The listing builds one solid part. Answer for the finished solid, in the listing's coordinates (mm). A direction names the side the tool comes from. Round coordinates to 2 decimals unless told otherwise and drop trailing zeros. Loops run counter-clockwise (first coordinate to the right, second up) from the corner with the lowest first, then second, coordinate; pieces in that order, holes last. Notation, with made-up numbers: (23.25, 47) -> (36.25, 47) arc R12 ccw to (36.25, 59) -> close; hole circle Ø8 at (51.5, 2). An arc over 180 degrees is marked (long way). Write each question's results on one line, items separated by ' | '. Start each with the question number.
from build123d import *

# Parameters (mm, degrees)
SKETCH1_W           = 44
SKETCH1_H           = 44
SKETCH1_R           = 2.25
SKETCH1_R_2         = 12
BOSS_EXTRUDE1_DEPTH = 5
SKETCH2_W           = 50
SKETCH2_H           = 44
SKETCH2_R           = 2.5
BOSS_EXTRUDE2_DEPTH = 5
BOSS_EXTRUDE3_DEPTH = 15
CHAMFER1_SIZE       = 7
CHAMFER2_SIZE       = 2
SKETCH4_W           = 50
SKETCH4_H           = 10.75
BOSS_EXTRUDE4_DEPTH = 10
CHAMFER3_SIZE       = 9
CHAMFER4_SIZE       = 2


with BuildPart() as part:
    # Sketch1 → Boss-Extrude1 (new body)
    with BuildSketch(Plane.XY):
        Rectangle(SKETCH1_W, SKETCH1_H)
        with Locations((15.5, 15.5)):
            Circle(SKETCH1_R, mode=Mode.SUBTRACT)
        with Locations((15.5, -15.5)):
            Circle(SKETCH1_R, mode=Mode.SUBTRACT)
        with Locations((-15.5, -15.5)):
            Circle(SKETCH1_R, mode=Mode.SUBTRACT)
        with Locations((-15.5, 15.5)):
            Circle(SKETCH1_R, mode=Mode.SUBTRACT)
        Circle(SKETCH1_R_2, mode=Mode.SUBTRACT)
    extrude(amount=BOSS_EXTRUDE1_DEPTH)

    # Sketch2 → Boss-Extrude2 (add)
    with BuildSketch(Plane.ZY.offset(22)):
        with Locations((25, 0)):
            Rectangle(SKETCH2_W, SKETCH2_H)
        with Locations(Location((44, 0, 0), (0, 0, 270))):
            Circle(SKETCH2_R, mode=Mode.SUBTRACT)
        with Locations(Location((24, 0, 0), (0, 0, 270))):
            Circle(SKETCH2_R, mode=Mode.SUBTRACT)
    extrude(amount=BOSS_EXTRUDE2_DEPTH)

    # Sketch3 → Boss-Extrude3 (add, symmetric)
    with BuildSketch(Plane(origin=(0, 0, 0), x_dir=(1, 0, 0), z_dir=(0, 1, 0))):
        Polygon((-14, -5), (-22, -13), (-22, -5), align=None)
    extrude(amount=BOSS_EXTRUDE3_DEPTH, both=True)

    # Chamfer1
    # the kernel refuses this chamfer: 7 mm, written as the material it takes off along each edge
    with BuildSketch(Plane(origin=(-1.270818641, -15, -7.729181359), x_dir=(-0.7068394360706735, -0.02749587661058637, -0.7068394360706736), z_dir=(-0.7071067811865477, 0, 0.7071067811865475))) as chamfer1_piece_1_section:
        Polygon((CHAMFER1_SIZE * 0.999621916911, -CHAMFER1_SIZE * 0.0274958766106), (-CHAMFER1_SIZE * 0.0274958766106, -CHAMFER1_SIZE * 0.999621916911), (0, 0), align=None)
    chamfer1_piece_1 = extrude(amount=47.317270331, mode=Mode.PRIVATE)
    chamfer1_piece_1 = split(chamfer1_piece_1, bisect_by=Plane(origin=(-22, -12.156184448, 8.014329888), z_dir=(1, 0, 0)), keep=Keep.TOP, mode=Mode.PRIVATE)
    chamfer1_piece_1 = split(chamfer1_piece_1, bisect_by=Plane(origin=(-19.249817179, -12.156184448, 5), z_dir=(0, 0, 1)), keep=Keep.TOP, mode=Mode.PRIVATE)
    add(chamfer1_piece_1, mode=Mode.SUBTRACT)
    with BuildSketch(Plane(origin=(-1.270818641, 15, -7.729181359), x_dir=(0.019442520806014066, -0.9996219169112968, 0.019442520806014073), z_dir=(-0.7071067811865477, 0, 0.7071067811865475))) as chamfer1_piece_2_section:
        Polygon((CHAMFER1_SIZE * 0.999621916911, -CHAMFER1_SIZE * 0.0274958766106), (-CHAMFER1_SIZE * 0.0274958766106, -CHAMFER1_SIZE * 0.999621916911), (0, 0), align=None)
    chamfer1_piece_2 = extrude(amount=47.317270331, mode=Mode.PRIVATE)
    chamfer1_piece_2 = split(chamfer1_piece_2, bisect_by=Plane(origin=(-22, 12.156184448, 8.014329888), z_dir=(1, 0, 0)), keep=Keep.TOP, mode=Mode.PRIVATE)
    chamfer1_piece_2 = split(chamfer1_piece_2, bisect_by=Plane(origin=(-19.249817179, 12.156184448, 5), z_dir=(0, 0, 1)), keep=Keep.TOP, mode=Mode.PRIVATE)
    add(chamfer1_piece_2, mode=Mode.SUBTRACT)

    # Chamfer2
    chamfer2_edges = [part.edges().sort_by_distance(p)[0] for p in [
        (-22, 2.5, 44),
        (-22, 2.5, 24),
    ]]
    chamfer(chamfer2_edges, length=CHAMFER2_SIZE)

    # Sketch4 → Boss-Extrude4 (add)
    with BuildSketch(Plane.ZY.offset(27)):
        with Locations((25, 16.625)):
            Rectangle(SKETCH4_W, SKETCH4_H)
        with Locations((25, -16.625)):
            Rectangle(SKETCH4_W, SKETCH4_H)
    extrude(amount=BOSS_EXTRUDE4_DEPTH)

    # Chamfer3
    chamfer3_edges = [part.edges().sort_by_distance(p)[0] for p in [
        (-37, -22, 25),
        (-37, 22, 25),
    ]]
    chamfer(chamfer3_edges, length=CHAMFER3_SIZE)

    # Chamfer4
    chamfer4_edges = [part.edges().sort_by_distance(p)[0] for p in [
        (13.25, 15.5, 5),
        (13.25, -15.5, 5),
        (-17.75, 15.5, 5),
        (-17.75, -15.5, 5),
    ]]
    chamfer(chamfer4_edges, length=CHAMFER4_SIZE)


solid = part.part
Item 1: The part is cut by section C-C, the plane x = 0. Give the vertices of the cut face in (y, z).
Item 2: For faces 5 (the flat face through (-32, -11.25, 25)), 6 (the flat face through (-37, 12, 25)), determine the directions among +Z, -Z, +X, -X, +Y, -Y from which every point of the face is accessible in a straight line to the end or side of a thin tool.
Item 3: Each of these flat-tipped pins is pushed along its axis until it touches: pin 1 Ø3 at (x, z) = (-30.5, 13.5) entering from +Y; pin 2 Ø10 at (x, y) = (-2.5, 7.5) entering from -Z; pin 3 Ø6 at (x, y) = (-15.5, -15.5) entering from +Z; pin 4 Ø2.5 at (x, y) = (15.5, -15.5) entering from +Z. Where does it stop, or does it pass through?
Item 4: The part is cut by section D-D, the plane y = 0. Give the vertices of the cut face in (x, z), plus the area to 3 significant figures.
Item 5: Straight lines are drawn through the part: L1, parallel to Y at x = -15.5, z = 0.85; L2, parallel to Z at x = -25, y = 0; L3, parallel to X at y = 13, z = 41. For each, find the intervals that lie inside material, in ascending order. Write a range as [from, to].
Item 6: Determine the mould class of faces 1 (the cylindrical face through (16.538, -17.496, 1.479)), 2 (the cylindrical face through (-14.462, 13.504, 1.479)), 3 (the flat face through (-33, 17, 25)), 4 (the flat face through (-32, 11.25, 25)) for opening direction X: +X half, -X half, draft (parallel to the pull), parting line (faces both ways), or undercut.
Item 7: The part is cut by section B-B, the plane y = 15.5. Give the vertices of the cut face in (x, z).
Item 8: The part is cut by section A-A, the plane x = 15.5. Give the vertices of the cut face in (y, z), plus the area to 3 significant figures.
Report:
1) outline: (-22, 0) -> (-12, 0) -> (-12, 5) -> (-22, 5) -> close; (12, 0) -> (22, 0) -> (22, 5) -> (12, 5) -> close
2) face 5: +Z, -Z, -X | face 6: +Z, -Z, -X, +Y, -Y
3) pin 1: stops at y = 21 | pin 2: stops at z = 0 | pin 3: stops at z = 3.75 | pin 4: passes through
4) outline: (-27, 0) -> (-12, 0) -> (-12, 5) -> (-14, 5) -> (-22, 13) -> (-22, 19.5) -> (-24, 21.5) -> (-27, 21.5) -> close; (-27, 26.5) -> (-24, 26.5) -> (-22, 28.5) -> (-22, 39.5) -> (-24, 41.5) -> (-27, 41.5) -> close; (-27, 46.5) -> (-24, 46.5) -> (-22, 48.5) -> (-22, 50) -> (-27, 50) -> close; (12, 0) -> (22, 0) -> (22, 5) -> (12, 5) -> close | area: 324 mm2
5) L1: y = [-22, -17.75], [-13.25, 13.25], [17.75, 22] | L2: z = [0, 21.5], [26.5, 41.5], [46.5, 50] | L3: x = [-37, -22]
6) face 1: undercut | face 2: undercut | face 3: -X half | face 4: draft
7) outline: (-34.5, 0) -> (-17.75, 0) -> (-17.75, 3) -> (-19.75, 5) -> (-22, 5) -> (-22, 50) -> (-34.5, 50) -> close; (-13.25, 0) -> (13.25, 0) -> (13.25, 3) -> (11.25, 5) -> (-11.25, 5) -> (-13.25, 3) -> close; (17.75, 0) -> (22, 0) -> (22, 5) -> (19.75, 5) -> (17.75, 3) -> close
8) outline: (-22, 0) -> (-17.75, 0) -> (-17.75, 3) -> (-19.75, 5) -> (-22, 5) -> close; (-13.25, 0) -> (13.25, 0) -> (13.25, 3) -> (11.25, 5) -> (-11.25, 5) -> (-13.25, 3) -> close; (17.75, 0) -> (22, 0) -> (22, 5) -> (19.75, 5) -> (17.75, 3) -> close | area: 167 mm2
